Autodesk Inventor part; units mm, degrees
ref_plane "YZ Plane" through (0, 0, 0) normal (1, 0, 0) x (0, 1, 0)
ref_plane "XZ Plane" through (0, 0, 0) normal (0, 1, 0) x (-1, 0, 0)
ref_plane "XY Plane" through (0, 0, 0) normal (0, 0, 1) x (1, 0, 0)
sketch "スケッチ1" plane through (0, 0, 0) normal (0, 0, 1) x (1, 0, 0)
  line L0 (0, 0) -> (54, 0)
  line L1 (54, 0) -> (54, 80)
  line L2 (54, 80) -> (0, 80)
  line L3 (0, 80) -> (0, 0)
  dimension "d0" = 54
  dimension "d1" = 80
extrude "押し出し1" add sketch "スケッチ1" along normal blind 5
sketch "スケッチ2" plane through (54, 0, 0) normal (1, 0, 0) x (0, 0, -1)
  line L0 (0, 0) -> (0, 80)
  line L1 (0, 80) -> (-5, 80)
  line L2 (-5, 0) -> (-5, 80)
  line L3 (0, 0) -> (-5, 0)
  line L4 (-5, 0) -> (-5, 80)
  line L5 (-5, 40) -> (0, 40) construction
  line L6 (0, 0) -> (0, 80)
  line L7 (-5, 75) -> (0, 75)
  line L8 (0, 75) -> (0, 42.5)
  line L9 (0, 42.5) -> (-5, 42.5)
  line L10 (-5, 42.5) -> (-5, 75)
  line L11 (-5, 5) -> (0, 5)
  line L12 (0, 5) -> (0, 37.5)
  line L13 (0, 37.5) -> (-5, 37.5)
  line L14 (-5, 37.5) -> (-5, 5)
  point P0 (0, 37.5)
  point P1 (-5, 37.5)
  point P2 (0, 5)
  point P3 (-5, 42.5)
  point P4 (0, 42.5)
  point P5 (0, 75)
  dimension "d4" = 5
  dimension "d5" = 5
extrude "押し出し2" add sketch "スケッチ2" along normal blind 2 contours L11 L2 L13 L0 | L9 L2 L7 L0
sketch "スケッチ3" plane through (0, 0, 0) normal (-1, 0, 0) x (0, 0, 1)
  line L0 (0, 42.5) -> (0, 75)
  line L1 (0, 75) -> (5, 75)
  line L2 (5, 75) -> (5, 42.5)
  line L3 (5, 42.5) -> (0, 42.5)
  line L4 (5, 37.5) -> (5, 5)
  line L5 (5, 5) -> (0, 5)
  line L6 (0, 5) -> (0, 37.5)
  line L7 (0, 37.5) -> (5, 37.5)
  point P0 (0, 0)
extrude "押し出し3" add sketch "スケッチ3" along normal blind 2
sketch "スケッチ4" plane through (0, 0, 5) normal (0, 0, 1) x (1, 0, 0)
  line L0 (54, 0) -> (54, 5)
  line L1 (54, 5) -> (56, 5)
  line L2 (56, 37.5) -> (56, 5)
  line L3 (54, 37.5) -> (56, 37.5)
  line L4 (54, 37.5) -> (54, 42.5)
  line L5 (54, 42.5) -> (56, 42.5)
  line L6 (56, 75) -> (56, 42.5)
  line L7 (54, 75) -> (56, 75)
  line L8 (54, 75) -> (54, 80)
  line L9 (54, 80) -> (0, 80)
  line L10 (0, 80) -> (0, 75)
  line L11 (0, 75) -> (-2, 75)
  line L12 (-2, 42.5) -> (-2, 75)
  line L13 (0, 42.5) -> (-2, 42.5)
  line L14 (0, 42.5) -> (0, 37.5)
  line L15 (0, 37.5) -> (-2, 37.5)
  line L16 (-2, 5) -> (-2, 37.5)
  line L17 (0, 5) -> (-2, 5)
  line L18 (0, 5) -> (0, 0)
  line L19 (0, 0) -> (54, 0)
  line L20 (54, 80) -> (0, 80)
  line L21 (27, 80) -> (27, 0) construction
  line L22 (0, 0) -> (54, 0)
  line L23 (5, 72) -> (49, 72)
  line L24 (49, 72) -> (49, 8)
  line L25 (49, 8) -> (5, 8)
  line L26 (5, 8) -> (5, 72)
  line L27 (0, 42.5) -> (0, 37.5)
  line L28 (0, 40) -> (54, 40) construction
  dimension "d10" = 8
  dimension "d11" = 5
extrude "押し出し4" cut sketch "スケッチ4" against normal through all contours L23 L24 L25 L26
fillet "フィレット1" radius 2 4 edges at (49, 72, 2.5) (5, 72, 2.5) (5, 8, 2.5) (49, 8, 2.5)
properties part number "foot_connect"
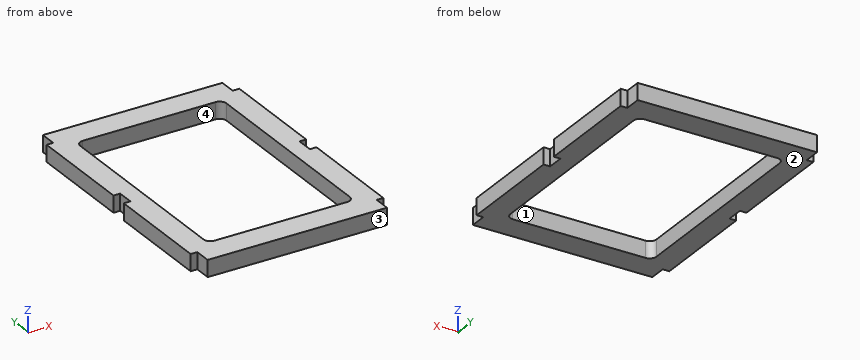
Build history of the part. All positions in model axes, mm. Face numbers are marked on the shaded views. A direction names the side the tool comes from. Coordinates: 2 decimals unless noted, no trailing zeros. Order: outer loops, then holes, each group sorted by start corner. A loop starts at its lowest first (then second) coordinate and runs counter-clockwise, first axis right, second up. Notation, with made-up numbers: (-3, 83) -> (10, 83) arc R19 cw to (10, 117) -> close; hole circle Ø10 at (72.25, 60). An arc over 180 degrees is marked (long way). Answer in a Markdown table with one row per item. Add a question column.
Q1. Band-saw the part on B-B, the plane y = 35.5. List the corners of the cut face in (x, z), then the cut area to 3 significant figures.
Q2. Wall check: line 1 along Y through (x, z) = (21, 4.4); line 2 along X through (y, z) = (66.5, 4.6); line 3 along X through (y, z) = (71.5, 1.75). Give the ranges that are in metal, low to high. Write a range as [from, to].
Q3. Which spindle directions (+Z, -Z, +X, -X, +Y, -Y) get a long thin tool onto all of the face, cutting with end or side? Do the marked faces 3 and 4. Say none if no direction does.
Q4. Drop flat-ended pins along their axis: pin 1 (1.5 mm diameter, centred on y = 40, z = 2.5, fed in from -X); pin 2 (0.6 mm diameter, centred on x = -1.5, z = 2, fed in from -Y); pin 3 (2 mm diameter, centred on x = 47, y = 11.5, fed in from +Z); pin 4 (1.5 mm diameter, centred on y = 39.5, z = 1.5, fed in from +X). Give the stop position or say it passes through.
Q5. Band-saw the part on C-C, the plane z = 2.05. List the corners of the cut face in (x, y).
Q6. Mould opens along X. For the marked faces 1 and 2 say: +X half, -X half, draft (parallel to the pull), parting line (faces both ways), or undercut.
Q7. Band-saw the part on A-A, the plane x = 8. List the corners of the cut face in (y, z), then the cut area to 3 significant figures.
Answers follow:
| question | item | result |
|---|---|---|
| 1 | outline | (-2, 0) -> (5, 0) -> (5, 5) -> (-2, 5) -> close; (49, 0) -> (56, 0) -> (56, 5) -> (49, 5) -> close |
| 1 | area | 70.0 mm^2 |
| 2 | line 1 | [0, 8], [72, 80] |
| 2 | line 2 | [-2, 5], [49, 56] |
| 2 | line 3 | [-2, 5.68], [48.32, 56] |
| 3 | face 3 | +Z, -Z, +X, -X, -Y |
| 3 | face 4 | +Z, -Z |
| 4 | pin 1 | x = 0 |
| 4 | pin 2 | y = 5 |
| 4 | pin 3 | through |
| 4 | pin 4 | x = 54 |
| 5 | outline | (-2, 5) -> (0, 5) -> (0, 0) -> (54, 0) -> (54, 5) -> (56, 5) -> (56, 37.5) -> (54, 37.5) -> (54, 42.5) -> (56, 42.5) -> (56, 75) -> (54, 75) -> (54, 80) -> (0, 80) -> (0, 75) -> (-2, 75) -> (-2, 42.5) -> (0, 42.5) -> (0, 37.5) -> (-2, 37.5) -> close; hole (5, 10) arc R2 ccw to (7, 8) -> (47, 8) arc R2 ccw to (49, 10) -> (49, 70) arc R2 ccw to (47, 72) -> (7, 72) arc R2 ccw to (5, 70) -> close |
| 6 | face 1 | undercut |
| 6 | face 2 | draft |
| 7 | outline | (0, 0) -> (8, 0) -> (8, 5) -> (0, 5) -> close; (72, 0) -> (80, 0) -> (80, 5) -> (72, 5) -> close |
| 7 | area | 80.0 mm^2 |
